from build123d import *

# Parameters (mm, degrees)
F0_W     = 63.5
F0_H     = 12.7
F0_W_2   = 76.2
F0_H_2   = 25.4
F0_W_3   = 53.3399905968
F0_W_4   = 63.5000094032
F1_DEPTH = 50.8


# Not quite as in the source:
# - ends of sketch curves that miss each other by under 0.0002 mm in the source are joined


with BuildPart() as f1:
    # F0 (on Top) → F1 (new body)
    with BuildSketch(Plane.XY):
        with Locations((-58.4199952984, 21.9910541385)):
            Rectangle(F0_W, F0_H)
        with BuildLine():
            Line((-102.8699952984, 15.6410541385), (-102.8699952984, -1.5747001893))
            Line((-102.8699952984, -1.5747001893), (-26.6699952984, -1.5747001893))
            Line((-26.6699952984, -1.5747001893), (-26.6699952984, 15.6410541385))
            Line((-26.6699952984, 15.6410541385), (-90.1699952984, 15.6410541385))
            Line((-90.1699952984, 15.6410541385), (-90.1699952984, 28.3410541385))
            ThreePointArc((-90.1699952984, 28.3410541385), (-99.1502514195, 24.6213102596), (-102.8699952984, 15.6410541385))
        make_face()
        with Locations((-64.7699952984, -14.2747001893)):
            Rectangle(F0_W_2, F0_H_2)
        with Locations((0, 21.9910541385)):
            Rectangle(F0_W_3, F0_H)
        with Locations((58.42, 21.9910541385)):
            Rectangle(F0_W_4, F0_H)
        with BuildLine():
            Line((90.1700047016, 15.6410541385), (26.6699952984, 15.6410541385))
            Line((26.6699952984, 15.6410541385), (26.6699952984, -1.5747001893))
            Line((26.6699952984, -1.5747001893), (102.8699952984, -1.5747001893))
            Line((102.8699952984, -1.5747001893), (102.8699952984, 15.6410541385))
            ThreePointArc((102.8699952984, 15.6410541385), (99.1502514195, 24.6213102596), (90.1699952984, 28.3410541385))
            Line((90.1699952984, 28.3410541385), (90.1700047016, 15.6410541385))
        make_face()
        with Locations((64.7699952984, -14.2747001893)):
            Rectangle(F0_W_2, F0_H_2)
    extrude(amount=F1_DEPTH)


solid = f1.part
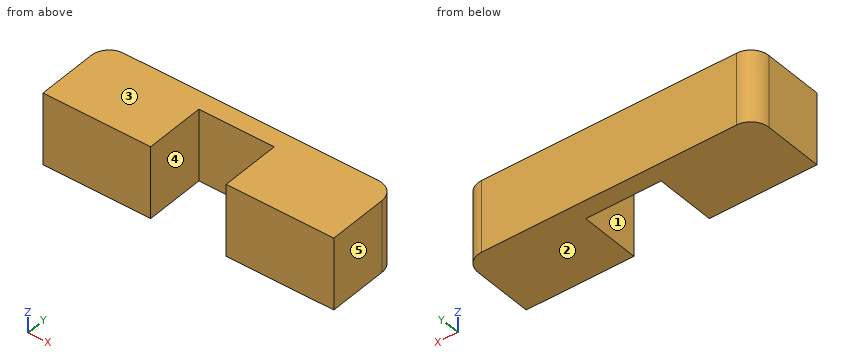
Build history of the part. All positions in model axes, mm. Face numbers are marked on the shaded views. A direction names the side the tool comes from. Give positions to 0.01 mm unless a question says otherwise; leave off trailing zeros. Order: outer loops, then holes, each group sorted by start corner. A loop starts at its lowest first (then second) coordinate and runs counter-clockwise, first axis right, second up. Notation, with made-up numbers: M 27,67 L 86,67 A17 cw 86,98 Z; hole C 68,-2 d11. An arc over 180 degrees is marked long. Use one line per item in the form item = value.
1) Saw through at A-A (y = -5.5). Give the cut face in (x, z).
Calculated:
outline = M -102.87,0 L -26.67,0 L -26.67,50.8 L -102.87,50.8 Z; M 26.67,0 L 102.87,0 L 102.87,50.8 L 26.67,50.8 Z
2) Saw through at B-B (z = 22). Give the cut face in (x, y).
Calculated:
outline = M -102.87,-26.97 L -26.67,-26.97 L -26.67,15.64 L 26.67,15.64 L 26.67,-26.97 L 102.87,-26.97 L 102.87,15.64 A12.7 ccw 90.17,28.34 L -90.17,28.34 A12.7 ccw -102.87,15.64 Z
3) Tool access for the marked faces 1 and 2: list every direction of +Z, -Z, +X, -X, +Y, -Y with a clear straight run to the whole face (end or side of a thin tool).
Calculated:
face_1 = +Z, -Z, -Y
face_2 = -Z, +X, -X, +Y, -Y
4) Drop flat-ended pins along their axis: pin 1 (1 mm diameter, centred on x = 22, z = 41, fed in from -Y); pin 2 (3 mm diameter, centred on y = 22, z = 6.5, fed in from +X). Give the stop position or say it passes through.
Calculated:
pin_1 = 15.64
pin_2 = 101.9
5) Two-plate mould, pull along X, no slides. Class the marked faces 3, 4 and 5: released by +X, released by -X, zero draft, split by the parting line, or undercut.
Calculated:
face_3 = zero draft
face_4 = undercut
face_5 = released by +X
6) Saw through at C-C (x = 1). Give the cut face in (y, z), plus the area to 3 significant figures.
Calculated:
outline = M 15.64,0 L 28.34,0 L 28.34,50.8 L 15.64,50.8 Z
area = 645 mm2
7) Probe probe 1 along X at (y, z) = (-12.5, 9.5); probe 2 along X at (y, z) = (16.5, 48); probe 3 along Y at (x, z) = (1, 25). List the from-to ranges inside material, lowest first.
Calculated:
probe_1 = -102.87 to -26.67, 26.67 to 102.87
probe_2 = -102.84 to 102.84
probe_3 = 15.64 to 28.34
